```python
from build123d import *

# Parameters (mm, degrees)
BOSS_EXTRUDE3_DEPTH = 30


with BuildPart() as part:
    # Sketch1 → Boss-Extrude3 (new body)
    with BuildSketch(Plane(origin=(0, 0, 0), x_dir=(1, 0, 0), z_dir=(0, 1, 0))):
        with BuildLine():
            Line((0, -25), (0, -32.168320657))
            ThreePointArc((0, -32.168320657), (-1.683972021, -32.124213487), (-3.36332613, -31.992012929))
            Line((-3.36332613, -31.992012929), (-17.67766953, -17.67766953))
            Line((-17.67766953, -17.67766953), (-22.746437676, -22.746437676))
            ThreePointArc((-22.746437676, -22.746437676), (-23.905997232, -21.524501161), (-25, -20.243538572))
            Line((-25, -20.243538572), (-25, 0))
            Line((-25, 0), (-32.168320657, 0))
            ThreePointArc((-32.168320657, 0), (-32.124213487, 1.683972021), (-31.992012929, 3.36332613))
            Line((-31.992012929, 3.36332613), (-17.67766953, 17.67766953))
            Line((-17.67766953, 17.67766953), (-22.746437676, 22.746437676))
            ThreePointArc((-22.746437676, 22.746437676), (-21.524501161, 23.905997232), (-20.243538572, 25))
            Line((-20.243538572, 25), (0, 25))
            Line((0, 25), (0, 32.168320657))
            ThreePointArc((0, 32.168320657), (1.683972021, 32.124213487), (3.36332613, 31.992012929))
            Line((3.36332613, 31.992012929), (17.67766953, 17.67766953))
            Line((17.67766953, 17.67766953), (22.746437676, 22.746437676))
            ThreePointArc((22.746437676, 22.746437676), (23.905997232, 21.524501161), (25, 20.243538572))
            Line((25, 20.243538572), (25, 0))
            Line((25, 0), (32.168320657, 0))
            ThreePointArc((32.168320657, 0), (32.124213487, -1.683972021), (31.992012929, -3.36332613))
            Line((31.992012929, -3.36332613), (17.67766953, -17.67766953))
            Line((17.67766953, -17.67766953), (22.746437676, -22.746437676))
            ThreePointArc((22.746437676, -22.746437676), (21.524501161, -23.905997232), (20.243538572, -25))
            Line((20.243538572, -25), (0, -25))
        make_face()
        with BuildLine():
            Line((-2, -16.860742714), (-2, -14.860742714))
            ThreePointArc((-2, -14.860742714), (0, 14.994721539), (2, -14.860742714))
            Line((2, -14.860742714), (2, -16.860742714))
            Line((2, -16.860742714), (-2, -16.860742714))
        make_face(mode=Mode.SUBTRACT)
    extrude(amount=BOSS_EXTRUDE3_DEPTH)


solid = part.part
```
Geometry check sheet. Reference: the model listing, model coordinates, mm. A direction names the side the tool comes from. Give positions to 0.01 mm unless a question says otherwise; leave off trailing zeros. Write each loop counter-clockwise with the first axis right and the second up, starting at its lowest first coordinate (ties: lowest second). Pieces come first, ordered by that corner, then holes.
1) Section check A-A, the plane y = 18.5. Record the boundary of the cut face in (x, z), and give its area (3 significant figures).
2) Material ranges on L1, parallel to Z at x = 20, y = 25.75; L2, parallel to Z at x = 11, y = 12.25; L3, parallel to X at y = 10, z = -18, recorded low to high.
3) Access from +Z, -Z, +X, -X, +Y, -Y to the whole of each face (thin tool, end or side, straight path). Record for faces 4 (the flat face through (29, 15, 0)), 5 (the flat face through (0, 15, 29)), 6 (the flat face through (-20, 15, 20)), 7 (the flat face through (0, 15, 16.861)).
4) Section check C-C, the plane z = -18.5. Record the boundary of the cut face in (x, y).
5) Gauge pin test, flat ends, axial feed: pin 1 (6 mm diameter, centred on y = 22, z = 5, fed in from -X); pin 2 (8 mm diameter, centred on y = 13, z = 29.5, fed in from +X); pin 3 (6 mm diameter, centred on x = -22.5, y = 22, fed in from -Z). Record the tip position at first contact, or that the pin passes through.
6) Release check for a two-part mould opening along Z. For faces 1 (the flat face through (-29, 15, 0)), 2 (the flat face through (2, 15, 16)), 3 (the cylindrical face through (-21.54, 14.79, -23.89)) record: pulls with the +Z half, pulls with the -Z half, needs draft (parallel to the pull), parting line crosses it, or undercut.
7) Section check B-B, the plane x = 7.5. Record the boundary of the cut face in (y, z).
Computed:
1. outline: (-32.17, 0) arc R32.17 ccw to (-31.99, -3.36) - (-17.68, -17.68) - (-22.75, -22.75) arc R32.17 ccw to (-20.24, -25) - (0, -25) - (0, -32.17) arc R32.17 ccw to (3.36, -31.99) - (17.68, -17.68) - (22.75, -22.75) arc R32.17 ccw to (25, -20.24) - (25, 0) - (32.17, 0) arc R32.17 ccw to (31.99, 3.36) - (17.68, 17.68) - (22.75, 22.75) arc R32.17 ccw to (20.24, 25) - (0, 25) - (0, 32.17) arc R32.17 ccw to (-3.36, 31.99) - (-17.68, 17.68) - (-22.75, 22.75) arc R32.17 ccw to (-25, 20.24) - (-25, 0) - close; hole (-2, 14.86) arc R14.99 ccw (long way) to (2, 14.86) - (2, 16.86) - (-2, 16.86) - close
1. area: 1,740 mm2
2. L1: z = -20 to 15.36, 20 to 25
2. L2: z = -24.36 to -10.19, 10.19 to 25
2. L3: x = -18 to 17.36, 18 to 25
3. face 4: -Z, +X, +Y, -Y
3. face 5: +Z, +X, +Y, -Y
3. face 6: +Z, +Y, -Y
3. face 7: +Y, -Y
4. outline: (-18.5, 0) - (16.86, 0) - (16.86, 30) - (-18.5, 30) - close; (18.5, 0) - (25, 0) - (25, 30) - (18.5, 30) - close
5. pin 1: stops at x = -25
5. pin 2: stops at x = 0
5. pin 3: stops at z = -25
6. face 1: pulls with the +Z half
6. face 2: undercut
6. face 3: pulls with the -Z half
7. outline: (0, -27.86) - (30, -27.86) - (30, -12.98) - (0, -12.98) - close; (0, 12.98) - (30, 12.98) - (30, 25) - (0, 25) - close
